Geometry: final body of the model. Coordinates: model frame, mm. A direction names the side the tool comes from. Give positions to 0.01 mm unless a question says otherwise; leave off trailing zeros. Write each loop counter-clockwise with the first axis right and the second up, starting at its lowest first coordinate (ties: lowest second). Pieces come first, ordered by that corner, then holes.
Q1. Cut plane D-D on z = 24. Return the cut outline in (x, y).
Q2. Line query: L1, parallel to Z at x = -1.5, y = 1.65; L2, parallel to Z at x = 10.5, y = 1.5; L3, parallel to X at y = 2.25, z = 0. Output: solid intervals per line, ascending.
Q3. Cut plane C-C on y = 0.7. Return the cut outline in (x, z), plus the area to 3 significant figures.
Q4. Pin query (flat end, axial travel): pin 1 (0.9 mm diameter, centred on y = 1, z = -1.5, fed in from -X); pin 2 (0.9 mm diameter, centred on x = -0.5, y = 1.5, fed in from -Z); pin 3 (1.5 mm diameter, centred on x = -26, y = 1.5, fed in from -Z). Return the tip coordinate at first contact, or that it passes through.
Q5. Cut plane A-A on x = 0. Return the cut outline in (y, z).
Q6. Cut plane B-B on z = 0. Return the cut outline in (x, y), plus the area to 3 significant figures.
Q7. Reachability of faces 5 (the face through (15, 1, 0)), 6 (the face through (-6, 1, -10)), 7 (the face through (-11.32, 1.48, 22.6)), 8 (the face through (19, 1, -25)) from +Z, -Z, +X, -X, +Y, -Y: full face, straight path, thin tool, end or side. Return the list, or none.
Q8. Draft query along Z for faces 1 (the face through (-12.409, 1.479, 13.395)), 2 (the face through (-26, 1, -19)), 3 (the face through (25, 1, 19)), 4 (the face through (-11, 1, 6)). Return one class per face: pulls with the +Z half, pulls with the -Z half, needs draft (parallel to the pull), parting line crosses it, or undercut.
```python
from build123d import *

# Parameters (mm, degrees)
SKETCH1_W           = 9
SKETCH1_H           = 2.5
SKETCH1_W_2         = 12
SKETCH1_H_2         = 9
SKETCH1_H_3         = 12
SKETCH1_R           = 3.6
SKETCH1_W_3         = 2.5
BOSS_EXTRUDE2_DEPTH = 3


with BuildPart() as part:
    # Sketch1 → Boss-Extrude2 (new body)
    # profile 1 of 13: a face of its own
    with BuildSketch(Plane(origin=(0, 0, 0), x_dir=(1, 0, 0), z_dir=(0, 1, 0))):
        Polygon((-6, 6), (-21, 19), (-21, 16.5), (-30, 16.5), (-15, 6), align=None)
    # profile 2 of 13: a face of its own
    with BuildSketch(Plane(origin=(0, 0, 0), x_dir=(1, 0, 0), z_dir=(0, 1, 0))):
        with Locations((-25.5, 17.75)):
            Rectangle(SKETCH1_W, SKETCH1_H)
    # profile 3 of 13: a face of its own
    with BuildSketch(Plane(origin=(0, 0, 0), x_dir=(1, 0, 0), z_dir=(0, 1, 0))):
        with Locations((0, 10.5)):
            Rectangle(SKETCH1_W_2, SKETCH1_H_2)
    # profile 4 of 13: a face of its own
    with BuildSketch(Plane(origin=(0, 0, 0), x_dir=(1, 0, 0), z_dir=(0, 1, 0))):
        with Locations((-10.5, 0)):
            Rectangle(SKETCH1_W, SKETCH1_H_3)
    # profile 5 of 13: a face of its own
    with BuildSketch(Plane(origin=(0, 0, 0), x_dir=(1, 0, 0), z_dir=(0, 1, 0))):
        Rectangle(SKETCH1_W_2, SKETCH1_H_3)
        with Locations(Location((0, 0, 0), (0, 0, 270))):
            Circle(SKETCH1_R, mode=Mode.SUBTRACT)
    # profile 6 of 13: a face of its own
    with BuildSketch(Plane(origin=(0, 0, 0), x_dir=(1, 0, 0), z_dir=(0, 1, 0))):
        with Locations((10.5, 0)):
            Rectangle(SKETCH1_W, SKETCH1_H_3)
    # profile 7 of 13: a face of its own
    with BuildSketch(Plane(origin=(0, 0, 0), x_dir=(1, 0, 0), z_dir=(0, 1, 0))):
        with Locations((0, -10.5)):
            Rectangle(SKETCH1_W_2, SKETCH1_H_2)
    # profile 8 of 13: a face of its own
    with BuildSketch(Plane(origin=(0, 0, 0), x_dir=(1, 0, 0), z_dir=(0, 1, 0))):
        Polygon((-6, -15), (-6, -6), (-19, -21), (-16.5, -21), (-16.5, -30), align=None)
    # profile 9 of 13: a face of its own
    with BuildSketch(Plane(origin=(0, 0, 0), x_dir=(1, 0, 0), z_dir=(0, 1, 0))):
        with Locations((-17.75, -25.5)):
            Rectangle(SKETCH1_W_3, SKETCH1_H_2)
    # profile 10 of 13: a face of its own
    with BuildSketch(Plane(origin=(0, 0, 0), x_dir=(1, 0, 0), z_dir=(0, 1, 0))):
        Polygon((15, -6), (6, -6), (21, -19), (21, -16.5), (30, -16.5), align=None)
    # profile 11 of 13: a face of its own
    with BuildSketch(Plane(origin=(0, 0, 0), x_dir=(1, 0, 0), z_dir=(0, 1, 0))):
        with Locations((25.5, -17.75)):
            Rectangle(SKETCH1_W, SKETCH1_H)
    # profile 12 of 13: a face of its own
    with BuildSketch(Plane(origin=(0, 0, 0), x_dir=(1, 0, 0), z_dir=(0, 1, 0))):
        Polygon((6, 15), (6, 6), (19, 21), (16.5, 21), (16.5, 30), align=None)
    # profile 13 of 13: a face of its own
    with BuildSketch(Plane(origin=(0, 0, 0), x_dir=(1, 0, 0), z_dir=(0, 1, 0))):
        with Locations((17.75, 25.5)):
            Rectangle(SKETCH1_W_3, SKETCH1_H_2)
    extrude(amount=BOSS_EXTRUDE2_DEPTH)


solid = part.part
```
Data:
1. outline: (-19, 0) - (-12.3, 0) - (-12.3, 3) - (-19, 3) - close
2. L1: z = -15 to -3.27, 3.27 to 15
2. L2: z = -21.43 to -11.19, -6 to 9.9
2. L3: x = -15 to -3.6, 3.6 to 15
3. outline: (-30, -19) - (-21, -19) - (-6, -6) - (-6, -15) - (6, -15) - (16.5, -30) - (19, -30) - (19, -21) - (6, -6) - (15, -6) - (15, 6) - (30, 16.5) - (30, 19) - (21, 19) - (6, 6) - (6, 15) - (-6, 15) - (-16.5, 30) - (-19, 30) - (-19, 21) - (-6, 6) - (-15, 6) - (-15, -6) - (-30, -16.5) - close; hole circle Ø7.2 at (0, 0)
3. area: 1,080 mm2
4. pin 1: stops at x = -15
4. pin 2: stops at z = -15
4. pin 3: stops at z = -19
5. outline: (0, -15) - (3, -15) - (3, -3.6) - (0, -3.6) - close; (0, 3.6) - (3, 3.6) - (3, 15) - (0, 15) - close
6. outline: (-15, 0) - (-3.6, 0) - (-3.6, 3) - (-15, 3) - close; (3.6, 0) - (15, 0) - (15, 3) - (3.6, 3) - close
6. area: 68.4 mm2
7. face 5: +X, +Y, -Y
7. face 6: -Z, +Y, -Y
7. face 7: +Z, +Y, -Y
7. face 8: -Z, +X, +Y, -Y
8. face 1: undercut
8. face 2: pulls with the -Z half
8. face 3: pulls with the +Z half
8. face 4: undercut
